```python
from build123d import *

# Parameters (mm, degrees)
F1_DEPTH = 774.7
F2_W     = 304.8
F2_H     = 158.75
F2_R     = 15.875
F2_W_2   = 203.2
F2_W_3   = 88.9
F2_H_2   = 558.8
F2_R_2   = 14.2875
F3_DEPTH = 25.4
F6_DEPTH = 12.7


with BuildPart() as f1:
    # F0 (on Right) → F1 (new body, symmetric)
    with BuildSketch(Plane.YZ):
        with BuildLine():
            Line((0, 209.55), (-330.2, 209.55))
            ThreePointArc((-330.2, 209.55), (-352.6506403027, 200.2506403027), (-361.95, 177.8))
            Line((-361.95, 177.8), (-361.95, -177.8))
            ThreePointArc((-361.95, -177.8), (-367.5296158184, -191.2703841816), (-381, -196.85))
            Line((-381, -196.85), (-488.95, -196.85))
            Line((-488.95, -196.85), (-488.95, -209.55))
            Line((-488.95, -209.55), (-381, -209.55))
            ThreePointArc((-381, -209.55), (-358.5493596973, -200.2506403027), (-349.25, -177.8))
            Line((-349.25, -177.8), (-349.25, 177.8))
            ThreePointArc((-349.25, 177.8), (-343.6703841816, 191.2703841816), (-330.2, 196.85))
            Line((-330.2, 196.85), (0, 196.85))
            Line((0, 196.85), (330.2, 196.85))
            ThreePointArc((330.2, 196.85), (343.6703841816, 191.2703841816), (349.25, 177.8))
            Line((349.25, 177.8), (349.25, -177.8))
            ThreePointArc((349.25, -177.8), (358.5493596973, -200.2506403027), (381, -209.55))
            Line((381, -209.55), (488.95, -209.55))
            Line((488.95, -209.55), (488.95, -196.85))
            Line((488.95, -196.85), (381, -196.85))
            ThreePointArc((381, -196.85), (367.5296158184, -191.2703841816), (361.95, -177.8))
            Line((361.95, -177.8), (361.95, 177.8))
            ThreePointArc((361.95, 177.8), (352.6506403027, 200.2506403027), (330.2, 209.55))
            Line((330.2, 209.55), (0, 209.55))
        make_face()
    extrude(amount=F1_DEPTH, both=True)

    # F2 (on face) → F3 (join)
    with BuildSketch(Plane.XY.offset(209.55)):
        with Locations((-341.376, -244.475)):
            Rectangle(F2_W, F2_H)
        with Locations((-398.526, -260.35)):
            Circle(F2_R, mode=Mode.SUBTRACT)
        with Locations((255.524, -244.475)):
            Rectangle(F2_W_2, F2_H)
        with Locations((261.874, -260.35)):
            Circle(F2_R, mode=Mode.SUBTRACT)
        with Locations((255.524, 244.475)):
            Rectangle(F2_W_2, F2_H)
        with Locations((261.874, 260.35)):
            Circle(F2_R, mode=Mode.SUBTRACT)
        with Locations((-341.376, 244.475)):
            Rectangle(F2_W, F2_H)
        with Locations((-398.526, 260.35)):
            Circle(F2_R, mode=Mode.SUBTRACT)
        with Locations((449.326, 0)):
            Rectangle(F2_W_3, F2_H_2)
        with Locations((449.072, -190.5)):
            Circle(F2_R_2, mode=Mode.SUBTRACT)
        with Locations((449.072, 190.5)):
            Circle(F2_R_2, mode=Mode.SUBTRACT)
        with Locations((722.122, 0)):
            Rectangle(F2_W_3, F2_H_2)
        with Locations((722.376, -190.5)):
            Circle(F2_R_2, mode=Mode.SUBTRACT)
        with Locations((722.376, 190.5)):
            Circle(F2_R_2, mode=Mode.SUBTRACT)
    extrude(amount=F3_DEPTH)

    # F5 (on offset) → F6 (join)
    with BuildSketch(Plane.YZ.offset(596.9)):
        Polygon((330.2, 196.85), (-330.2, 196.85), (-349.25, 177.8), (-349.25, -209.55), (349.25, -209.55), (349.25, 177.8), align=None)
    extrude(amount=-F6_DEPTH)


solid = f1.part
```
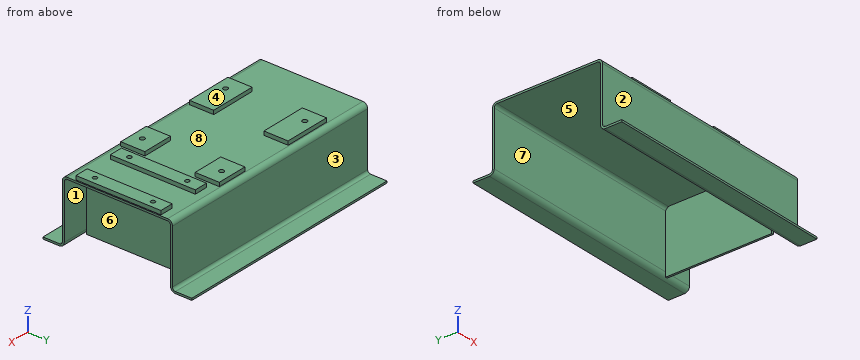
Read the model definition and answer for the solid it produces. Units are mm, in the model's axes. Face numbers are marked on the shaded views. A direction names the side the tool comes from. Round coordinates to 2 decimals unless told otherwise and drop trailing zeros. Write each loop counter-clockwise with the first axis right and the second up, starting at its lowest first coordinate (ties: lowest second). Pieces come first, ordered by that corner, then holes. Notation, with made-up numbers: (61, 42) - (66, 42) arc R14 cw to (66, 51) - close; hole circle Ø2 at (74.5, 51.5). An arc over 180 degrees is marked (long way). Use CSV: the item, a comma, the result in double quotes.
Q1. Find section C-C, the plane x = -569. Write down the section's boundary in (y, z).
Values:
outline,"(-488.95, -209.55) - (-381, -209.55) arc R31.75 ccw to (-349.25, -177.8) - (-349.25, 177.8) arc R19.05 cw to (-330.2, 196.85) - (330.2, 196.85) arc R19.05 cw to (349.25, 177.8) - (349.25, -177.8) arc R31.75 ccw to (381, -209.55) - (488.95, -209.55) - (488.95, -196.85) - (381, -196.85) arc R19.05 cw to (361.95, -177.8) - (361.95, 177.8) arc R31.75 ccw to (330.2, 209.55) - (-330.2, 209.55) arc R31.75 ccw to (-361.95, 177.8) - (-361.95, -177.8) arc R19.05 cw to (-381, -196.85) - (-488.95, -196.85) - close"
Q2. A tool of negligible diameter and unlimited length cuts with its end or side. For the marked faces 1, 2, 3, 4 and 5, from which of +Z, -Z, +X, -X, +Y, -Y can it reach the whole face along a straight path? Write none if from no direction.
Values:
face 1,"-Z, +X"
face 2,"+Z, +X, -X, -Y"
face 3,"+Z, +X, -X, +Y"
face 4,"+Z, +X, -X, +Y, -Y"
face 5,"-Z, -X"
Q3. Find section A-A, the plane z = -2.5. Write down the section's boundary in (x, y), then the cut area to 3 significant figures.
Values:
outline,"(-774.7, -361.95) - (774.7, -361.95) - (774.7, -349.25) - (596.9, -349.25) - (596.9, 349.25) - (774.7, 349.25) - (774.7, 361.95) - (-774.7, 361.95) - (-774.7, 349.25) - (584.2, 349.25) - (584.2, -349.25) - (-774.7, -349.25) - close"
area,"48,200 mm²"
Q4. Determine the mould class of the marked faces 6, 7 and 8 for opening direction X: +X half, -X half, draft (parallel to the pull), parting line (faces both ways), or undercut.
Values:
face 6,"+X half"
face 7,"draft"
face 8,"undercut"
Q5. Find section B-B, the plane y = 57.5. Write down the section's boundary in (x, z), then the cut area to 3 significant figures.
Values:
outline,"(-774.7, 196.85) - (584.2, 196.85) - (584.2, -209.55) - (596.9, -209.55) - (596.9, 196.85) - (774.7, 196.85) - (774.7, 209.55) - (766.57, 209.55) - (766.57, 234.95) - (677.67, 234.95) - (677.67, 209.55) - (493.78, 209.55) - (493.78, 234.95) - (404.88, 234.95) - (404.88, 209.55) - (-774.7, 209.55) - close"
area,"29,400 mm²"
Q6. Straight lines are drawn through the part: line 1 along Y through (x, z) = (713, 7); line 2 along X through (y, z) = (-337.5, 37); line 3 along Z through (x, y) = (-457.5, 108). For each, find the intervals that lie inside material, in ascending order.
Values:
line 1,"y = -361.95 to -349.25, 349.25 to 361.95"
line 2,"x = 584.2 to 596.9"
line 3,"z = 196.85 to 209.55"
Q7. Each of these flat-tipped pins is pushed along its axis until it touches: pin 1 Ø8.5 at (x, y) = (452.5, 184.5) entering from +Z; pin 2 Ø20.5 at (y, z) = (72, 225) entering from -X; pin 3 Ø7.5 at (x, z) = (717, 222.5) entering from +Y. Where does it stop, or does it pass through?
Values:
pin 1,"stops at z = 209.55"
pin 2,"stops at x = 404.88"
pin 3,"stops at y = 279.4"
